Source: CAD feature listing. Evaluate the final solid. Frame: model axes, mm. Round coordinates to 2 decimals unless told otherwise and drop trailing zeros. Loops run counter-clockwise (first coordinate to the right, second up) from the corner with the lowest first, then second, coordinate; pieces in that order, holes last. Notation, with made-up numbers: M 8.25,34.5 L 41.25,34.5 A19 cw 41.25,59.5 Z; hole C -18,-31.5 d8. An arc over 180 degrees is marked long. Answer as a JSON object with one key per item and string values.
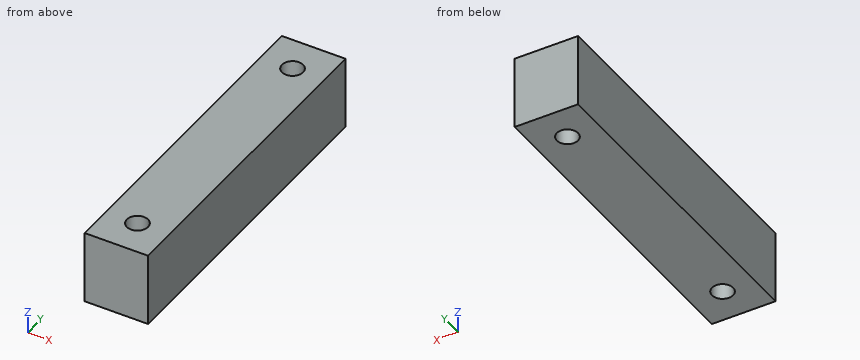
Autodesk Inventor part; units mm, degrees
ref_plane "YZ Plane" through (0, 0, 0) normal (1, 0, 0) x (0, 1, 0)
ref_plane "XZ Plane" through (0, 0, 0) normal (0, 1, 0) x (-1, 0, 0)
ref_plane "XY Plane" through (0, 0, 0) normal (0, 0, 1) x (1, 0, 0)
ref_plane "Plan de construction1" through (0, 0, 0) normal (0, 0, 1) x (1, 0, 0)
sketch "Esquisse1" plane through (0, 0, 0) normal (0, 0, 1) x (1, 0, 0)
  circle A0 centre (36.4553, 35.5016) radius 2.25
  line L0 (29.7194, 25.7651) -> (43.1911, 25.7651)
  line L1 (43.1911, 25.7651) -> (43.1911, 43.0016)
  line L2 (43.1911, 43.0016) -> (29.7194, 43.0016)
  line L3 (29.7194, 43.0016) -> (29.7194, 25.7651)
  circle A1 centre (36.4553, -19.4032) radius 2.25
  circle A2 centre (36.4553, 35.5016) radius 2.25
  circle A3 centre (25.0518, -6.7548) radius 2.15
  circle A4 centre (25.0518, 23.2452) radius 2.15
  line L4 (43.1911, 43.0016) -> (43.1911, -26.9032)
  line L5 (29.7194, 43.0016) -> (43.1911, 43.0016)
  line L6 (29.7194, 28.2452) -> (29.7194, 43.0016)
  line L7 (29.7194, 28.2452) -> (19.7194, 28.2452)
  line L8 (19.7194, 28.2452) -> (19.7194, 19.2452)
  line L9 (19.7194, 19.2452) -> (38.63, 19.2452)
  line L10 (38.63, 19.2452) -> (38.63, -2.9032)
  line L11 (38.63, -2.9032) -> (19.7194, -2.9032)
  line L12 (19.7194, -2.9032) -> (19.7194, -11.9032)
  line L13 (19.7194, -11.9032) -> (29.7194, -11.9032)
  line L14 (29.7194, -26.9032) -> (29.7194, -11.9032)
  line L15 (43.1911, -26.9032) -> (29.7194, -26.9032)
  line L16 (43.1911, 43.0016) -> (29.7194, 43.0016)
  line L17 (29.7194, 43.0016) -> (29.7194, -26.9032)
  line L18 (29.7194, -26.9032) -> (43.1911, -26.9032)
  line L19 (43.1911, -26.9032) -> (43.1911, 43.0016)
  point P0 (0, 0)
extrude "Extrusion1" add sketch "Esquisse1" along normal blind 15.5 contours L3 L2 L1 L0 | L0 L4 L15 L14 L17 L11 L10 L9 | L9 L10 L11 L17
properties part number "tg"
Item 1: Section A-A on x = 37.25. Return the cut outline in (y, z), then the cut area to 3 significant figures.
Answer sheet:
{"outline": "M -26.9,0 L -21.51,0 L -21.51,15.5 L -26.9,15.5 Z; M -17.3,0 L 33.4,0 L 33.4,15.5 L -17.3,15.5 Z; M 37.61,0 L 43,0 L 43,15.5 L 37.61,15.5 Z", "area": "953 mm²"}
Item 2: Line query: probe 1 along X at (y, z) = (-21, 2); probe 2 along X at (y, z) = (35, 7). Output: solid intervals per line, ascending. Write a range as from..to.
Answer sheet:
{"probe 1": "x = 29.72..34.87, 38.04..43.19", "probe 2": "x = 29.72..34.26, 38.65..43.19"}
Item 3: Section B-B on z = 6.5. Return the cut outline in (x, y).
Answer sheet:
{"outline": "M 29.72,-26.9 L 43.19,-26.9 L 43.19,43 L 29.72,43 Z; hole C 36.46,-19.4 d4.5; hole C 36.46,35.5 d4.5"}
